Autodesk Inventor part; units mm, degrees
ref_plane "YZ Plane" through (0, 0, 0) normal (1, 0, 0) x (0, 1, 0)
ref_plane "XZ Plane" through (0, 0, 0) normal (0, 1, 0) x (-1, 0, 0)
ref_plane "XY Plane" through (0, 0, 0) normal (0, 0, 1) x (1, 0, 0)
sketch "Esboço1" plane through (0, 0, 0) normal (0, 0, 1) x (1, 0, 0)
  line L0 (-17, 15) -> (17, 15)
  line L1 (17, 15) -> (17, -15)
  line L2 (17, -15) -> (-17, -15)
  line L3 (-17, -15) -> (-17, 15)
  line L4 (-17, 15) -> (17, -15) construction
  line L5 (17, 15) -> (-17, -15) construction
  point P0 (0, 0)
  dimension "d0" = 34
  dimension "d1" = 30
extrude "Extrusão1" add sketch "Esboço1" along normal blind 30
sketch "Esboço2" plane through (0, 0, 30) normal (0, 0, 1) x (1, 0, 0)
  circle A0 centre (0, 0) radius 8 construction
  circle A1 centre (-0.0751, 7.9996) radius 1 construction
  circle A2 centre (0, 0) radius 8 construction
  circle A3 centre (-7.9996, -0.0751) radius 1 construction
  circle A4 centre (0, 0) radius 8 construction
  circle A5 centre (0.0751, -7.9996) radius 1 construction
  circle A6 centre (0, 0) radius 8 construction
  circle A7 centre (7.9996, 0.0751) radius 1 construction
  dimension "d4" = 16
  dimension "d5" = 2
  dimension "d8" = 360
hole "Furo1" at (-0.0751, 7.9996, 30) at (-7.9996, -0.0751, 30) at (7.9996, 0.0751, 30) at (0.0751, -7.9996, 30) direction (0, 0, -1) diameter 2.459 depth 8 tip angle 118
sketch "Esboço3" plane through (0, 0, 30) normal (0, 0, 1) x (1, 0, 0)
  circle A0 centre (0, 0) radius 5.25
  dimension "d17" = 10.5
hole "Furo2" at (0, 0, 30) direction (0, 0, -1) diameter 10.5 end through all
sketch "Esboço4" plane through (-17, 15, 0) normal (0, 1, 0) x (1, 0, 0)
  line L0 (0, 0) -> (0, -30) construction
  line L1 (0, -15) -> (34, -15) construction
  line L2 (34, 0) -> (34, -30) construction
  line L3 (18.1544, -30) -> (15.6954, -30) construction
  line L4 (16.9249, -30) -> (17, 0) construction
  line L5 (11.75, 0) -> (22.25, 0) construction
  circle A0 centre (4.9874, -5) radius 1 construction
  circle A1 centre (28.9875, -5) radius 1 construction
  circle A2 centre (28.9374, -25) radius 1 construction
  circle A3 centre (4.9374, -25) radius 1 construction
  dimension "d25" = 2
  dimension "d26" = 2
  dimension "d27" = 2
  dimension "d28" = 2
  dimension "d29" = 10
  dimension "d30" = 10
  dimension "d31" = 10
  dimension "d32" = 10
  dimension "d33" = 12
  dimension "d34" = 12
  dimension "d35" = 12
  dimension "d36" = 12
hole "Furo3" at (-12.0626, 15, 25) at (-12.0126, 15, 5) at (11.9875, 15, 5) at (11.9374, 15, 25) direction (0, -1, 0) diameter 3.242 depth 12 tip angle 118
equation "\"d30\" = d29"
equation "\"d31\" = d29"
equation "\"d32\" = d29"
equation "\"d34\" = d33"
equation "\"d35\" = d33"
equation "\"d36\" = d33"
properties part number "SuporteCastanhaTr8"
Model file for the job. Use its own axes, mm. A direction names the side the tool comes from. Give positions to 0.01 mm unless a question says otherwise; leave off trailing zeros. Write each loop counter-clockwise with the first axis right and the second up, starting at its lowest first coordinate (ties: lowest second). Pieces come first, ordered by that corner, then holes. Notation, with made-up numbers: (-5, -19) - (26, -19) arc R27 cw to (26, 18) - close; hole circle Ø2 at (32.25, -27). An arc over 180 degrees is marked (long way). One line per question, with ' | ' between items. Start each with the question number.
(1) Slice it at A-A on y = -1.75. Write the cut outline in (x, z).
(2) Slice it at C-C on z = 12.5. Write the cut outline in (x, y), plus the area to 3 significant figures.
(3) Pin check, flat tips, straight feed: P1, Ø2.5, axis at x = 11.99, z = 5, coming from the +Y side; P2, Ø3, axis at x = 11.94, z = 25, coming from the +Y side. Stop position of each tip, or through.
(4) Slice it at D-D on y = 10. Write the cut outline in (x, z).
(5) 3-axis set-ups, long thin cutter, end or side, ignore diameter. For faces 4 (the face through (-10.43, 8.92, 4.65)), 5 (the face through (17, 0, 15)), 6 (the face through (6.78, 0.24, 25.94)): which of +Z, -Z, +X, -X, +Y, -Y reach the whole face in a straight line?
(6) Slice it at B-B on x = 4.5. Write the cut outline in (y, z), plus the area to 3 significant figures.
(7) Wall check: line 1 along X through (y, z) = (10, 5); line 2 along Z through (x, y) = (-12, 8.5); line 3 along X through (y, z) = (11.75, 25). Give the ranges that are in metal, low to high. Write a range as from..to.
(8) Two-plate mould, pull along Y, no slides. Class faces 1 (the face through (-17, 0, 15)), 2 (the face through (11.713, 2.195, 4.939)), 3 (the face through (-1.6, -5, 14.8)): +Y half, -Y half, draft (parallel to the pull), parting line (faces both ways), or undercut.
Results below:
1) outline: (-17, 0) - (-4.95, 0) - (-4.95, 30) - (-17, 30) - close; (4.95, 0) - (17, 0) - (17, 30) - (4.95, 30) - close
2) outline: (-17, -15) - (17, -15) - (17, 15) - (-17, 15) - close; hole circle Ø10.5 at (0, 0) | area: 933 mm^2
3) P1: y = 2.78 | P2: y = 2.93
4) outline: (-17, 0) - (17, 0) - (17, 30) - (-17, 30) - close; hole circle Ø3.24 at (-12.06, 25); hole circle Ø3.24 at (-12.01, 5); hole circle Ø3.24 at (11.94, 25); hole circle Ø3.24 at (11.99, 5)
5) face 4: +Y | face 5: +Z, -Z, +X, +Y, -Y | face 6: +Z
6) outline: (-15, 0) - (-2.7, 0) - (-2.7, 30) - (-15, 30) - close; (2.7, 0) - (15, 0) - (15, 30) - (2.7, 30) - close | area: 738 mm^2
7) line 1: -17..-13.63, -10.39..10.37, 13.61..17 | line 2: 0..3.38, 6.62..23.38, 26.62..30 | line 3: -17..-13.68, -10.44..10.32, 13.56..17
8) face 1: draft | face 2: +Y half | face 3: undercut
